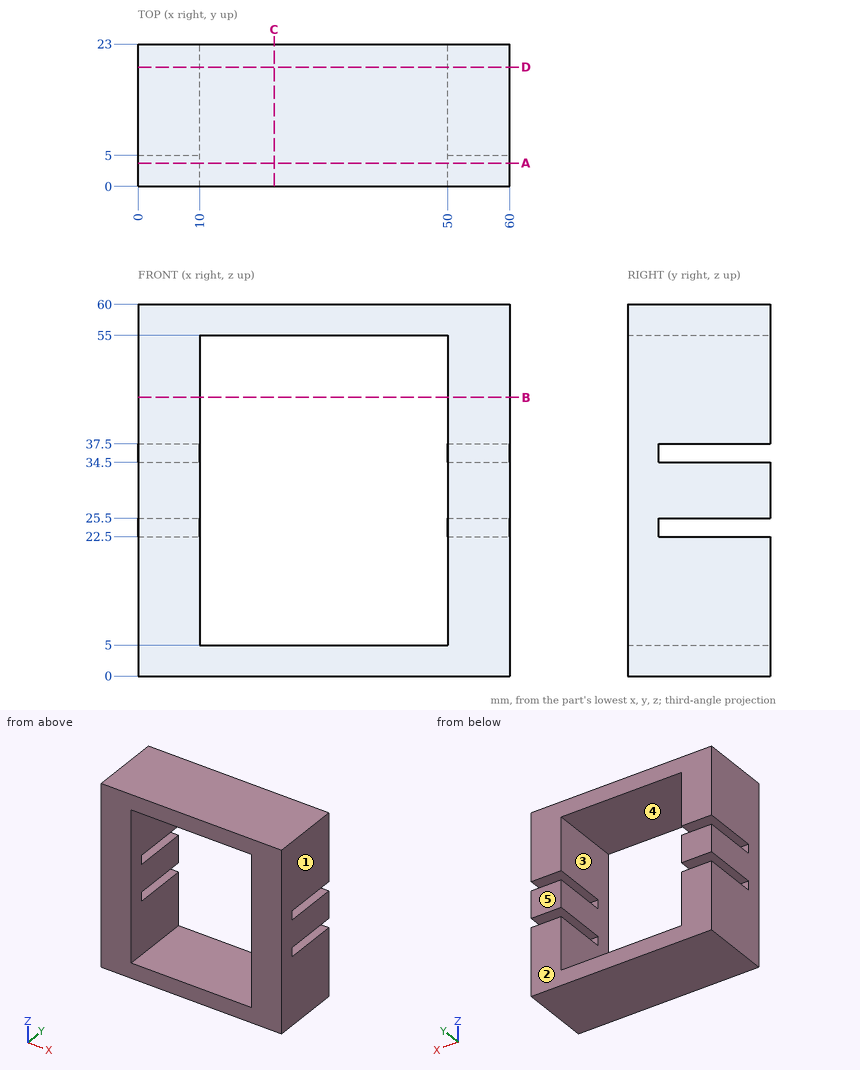
Geometry check sheet. Reference: drawing and pictorial views, mm from the part's lowest x, y, z. A direction names the side the tool comes from. Coordinates: 2 decimals unless noted, no trailing zeros. Order: outer loops, then holes, each group sorted by start corner. A loop starts at its lowest first (then second) coordinate and runs counter-clockwise, first axis right, second up. Notation, with made-up numbers: (12, 65) - (66, 65) arc R31 cw to (66, 101) - close; hole circle Ø2 at (54.5, 8). An arc over 180 degrees is marked (long way). One line per item, written item: value.
(1) Sectioned sample at C-C (x = 22). Enter the section's corners in (y, z).
Data:
outline: (0, 0) - (23, 0) - (23, 5) - (0, 5) - close; (0, 55) - (23, 55) - (23, 60) - (0, 60) - close
(2) Release check for a two-part mould opening along X. For the marked faces 1, 2 and 3 record: +X half, -X half, draft (parallel to the pull), parting line (faces both ways), or undercut.
Data:
face 1: +X half
face 2: draft
face 3: undercut
(3) Sectioned sample at B-B (z = 45). Enter the section's corners in (x, y), and give its area (3 significant figures).
Data:
outline: (0, 0) - (10, 0) - (10, 23) - (0, 23) - close; (50, 0) - (60, 0) - (60, 23) - (50, 23) - close
area: 460 mm^2
(4) Depth check by flat-ended pin: pin 1 Ø2.5 at (x, z) = (6.5, 24) entering from +Y. Enter the tip coordinate at first touch or a pass-through.
Data:
pin 1: stops at y = 5
(5) Sectioned sample at D-D (y = 19.25). Enter the section's corners in (x, z), and give its area (3 significant figures).
Data:
outline: (0, 0) - (60, 0) - (60, 22.5) - (50, 22.5) - (50, 5) - (10, 5) - (10, 22.5) - (0, 22.5) - close; (0, 25.5) - (10, 25.5) - (10, 34.5) - (0, 34.5) - close; (0, 37.5) - (10, 37.5) - (10, 55) - (50, 55) - (50, 37.5) - (60, 37.5) - (60, 60) - (0, 60) - close; (50, 25.5) - (60, 25.5) - (60, 34.5) - (50, 34.5) - close
area: 1,480 mm^2
(6) Access from +Z, -Z, +X, -X, +Y, -Y to the whole of each face (thin tool, end or side, straight path). Record for the marked faces 4 and 5.
Data:
face 4: +Y, -Y
face 5: +Z, -Z, +X, -X, +Y
(7) Thickness scan on probe 1 along Z at (x, y) = (3, 5.5); probe 2 along X at (y, z) = (6.75, 40.5); probe 3 along Z at (x, y) = (29, 19.5). Record the ranges inside material, lowest first. Write a range as from..to.
Data:
probe 1: z = 0..22.5, 25.5..34.5, 37.5..60
probe 2: x = 0..10, 50..60
probe 3: z = 0..5, 55..60
(8) Sectioned sample at A-A (y = 3.75). Enter the section's corners in (x, z), and give its area (3 significant figures).
Data:
outline: (0, 0) - (60, 0) - (60, 60) - (0, 60) - close; hole (10, 5) - (50, 5) - (50, 55) - (10, 55) - close
area: 1,600 mm^2
